For this review, use the dimensioned drawing (mm, ordinates from the lowest corner) and the shaded views. A direction names the side the tool comes from. Coordinates: 2 decimals unless noted, no trailing zeros. Write each loop counter-clockwise with the first axis right and the second up, starting at its lowest first coordinate (ties: lowest second). Pieces come first, ordered by that corner, then holes.
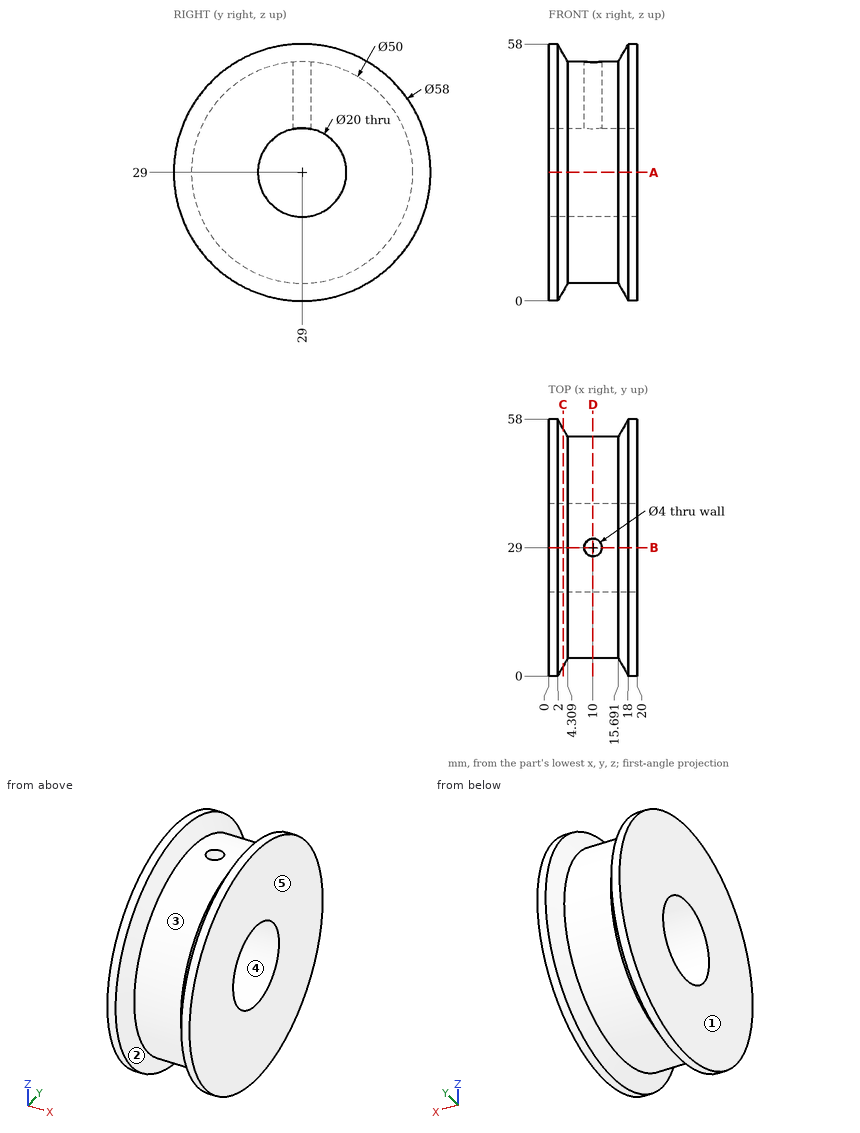
(1) Consider section C-C (x = 3.25). Give the boundary of the cut face in (y, z) (1 decimal), plus the area to 3 significant figures.
(2) For the marked faces 1 and 2, list the 3-axis set-ups (+Z, -Z, +X, -X, +Y, -Y) from which the entire face can be reached by the end or side of a thin tool; tool diameter is ignored.
(3) Wall thickness on line 1 (Z direction, x = 14, y = 29); line 2 (Z direction, x = 10, y = 29); line 3 (Y direction, x = 10, z = 46.25) (1 decimal): over which ranges is each line inside the solid? List them lowest first.
(4) Consider section B-B (y = 29). Give the boundary of the cut face in (x, z).
(5) Mouldability with a two-part tool opening along Z and no side actions: class the marked faces 3, 4 and 5 as +Z half, -Z half, draft (parallel to the pull), parting line (faces both ways), or undercut.
(6) Consider section D-D (x = 10). Give the boundary of the cut face in (y, z).
(7) Insertion check: pin 1 Ø4.5 at (x, y) = (10, 29) entering from +Z; pin 2 Ø4 at (x, z) = (6.5, 7) entering from -Y; pin 3 Ø3 at (x, y) = (15.5, 35) entering from +Z. Each pin has a flat end and moves straight along its axis. Give the tip position at first contact, or say it passes through.
(8) Consider section A-A (z = 29). Give the boundary of the cut face in (x, y).
Results:
1. outline: circle Ø53.7 at (29, 29); hole circle Ø20 at (29, 29)
1. area: 1,950 mm2
2. face 1: +Z, -Z, -X, +Y, -Y
2. face 2: none
3. line 1: z = 4 to 19, 39 to 54
3. line 2: z = 4 to 19
3. line 3: y = 10.9 to 27, 31 to 47.1
4. outline: (0, 0) - (2, 0) - (4.31, 4) - (15.69, 4) - (18, 0) - (20, 0) - (20, 19) - (0, 19) - close; (0, 39) - (8, 39) - (8, 54) - (4.31, 54) - (2, 58) - (0, 58) - close; (12, 39) - (20, 39) - (20, 58) - (18, 58) - (15.69, 54) - (12, 54) - close
5. face 3: parting line
5. face 4: undercut
5. face 5: draft
6. outline: (27, 38.8) - (27, 53.92) arc R25 ccw (long way) to (31, 53.92) - (31, 38.8) arc R10 cw (long way) to start
7. pin 1: stops at z = 54
7. pin 2: stops at y = 14
7. pin 3: stops at z = 55.62
8. outline: (0, 0) - (2, 0) - (4.31, 4) - (15.69, 4) - (18, 0) - (20, 0) - (20, 19) - (0, 19) - close; (0, 39) - (20, 39) - (20, 58) - (18, 58) - (15.69, 54) - (4.31, 54) - (2, 58) - (0, 58) - close
